Check sheet for the modelled part. Datum: model origin and axes. Units: mm. A direction names the side the tool comes from. Round coordinates to 2 decimals unless told otherwise and drop trailing zeros. Order: outer loops, then holes, each group sorted by start corner. A loop starts at its lowest first (then second) coordinate and runs counter-clockwise, first axis right, second up.
```python
from build123d import *

# Parameters (mm, degrees)
F0_W     = 21
F0_H     = 4
F0_R     = 26.5
F0_R_2   = 1
F1_DEPTH = 3
F2_DEPTH = 10
F4_R     = 1
F5_DEPTH = 37.501


with BuildPart() as f1:
    # F0 (on Front) → F1 (new body)
    with BuildSketch(Plane.XZ):
        with Locations((10.5, 9)):
            Rectangle(F0_W, F0_H)
        with Locations((-10.5, 9)):
            Rectangle(F0_W, F0_H)
        Circle(F0_R)
        with Locations((-16.334167, -16.334167)):
            Circle(F0_R_2, mode=Mode.SUBTRACT)
        with Locations((16.334167, -16.334167)):
            Circle(F0_R_2, mode=Mode.SUBTRACT)
        with Locations((-16.334167, 16.334167)):
            Circle(F0_R_2, mode=Mode.SUBTRACT)
        Polygon((21, 7), (0, 7), (-21, 7), (-21, 11), (0, 11), (21, 11), align=None, mode=Mode.SUBTRACT)
        with Locations((16.334167, 16.334167)):
            Circle(F0_R_2, mode=Mode.SUBTRACT)
    extrude(amount=F1_DEPTH)

    # F0 (on Front) → F2 (join)
    with BuildSketch(Plane.XZ):
        with Locations((10.5, 9)):
            Rectangle(F0_W, F0_H)
        with Locations((-10.5, 9)):
            Rectangle(F0_W, F0_H)
    extrude(amount=-F2_DEPTH)

    # F3: F1 across plane


with BuildPart() as f1_1:
    add(f1.part)
    add(f1.part.mirror(Plane.XY))

    # F4 (on face) → F5 (cut, through all)
    with BuildSketch(Plane.XY.offset(11)):
        with Locations((-12, 3)):
            Circle(F4_R)
        with Locations((12, 3)):
            Circle(F4_R)
    extrude(amount=-F5_DEPTH, mode=Mode.SUBTRACT)


solid = f1_1.part
```
Item 1: Go/stop test with flat-tipped pins: P1, Ø3, axis at x = 1.5, y = 2.5, coming from the +Z side; P2, Ø5, axis at x = 2.5, y = 6.5, coming from the -Z side; P3, Ø2, axis at y = 3, z = -9, coming from the +X side. Record where each tip stops, or that it passes through.
Answer:
P1: stops at z = 11
P2: stops at z = -11
P3: stops at x = 21
Item 2: Release check for a two-part mould opening along X. For faces 1 (the cylindrical face through (14.246, -1.479, 22.345)), 2 (the cylindrical face through (-15.41, -1.48, -16.72)), 3 (the flat face through (0, 5, -11)), 4 (the cylindrical face through (-13, 3, -9)) record: released by +X, released by -X, zero draft, split by the parting line, or undercut.
Answer:
face 1: split by the parting line
face 2: undercut
face 3: zero draft
face 4: undercut
Item 3: Sectioned sample at A-A (y = 7.25). Record the cut outline in (x, z), and give its area (3 significant figures).
Answer:
outline: (-21, -11) - (21, -11) - (21, -7) - (-21, -7) - close; (-21, 7) - (21, 7) - (21, 11) - (-21, 11) - close
area: 336 mm2
Item 4: Sectioned sample at C-C (x = -12). Record the cut outline in (y, z), and give its area (3 significant figures).
Answer:
outline: (-3, -23.63) - (0, -23.63) - (0, -11) - (2, -11) - (2, -7) - (0, -7) - (0, 7) - (2, 7) - (2, 11) - (0, 11) - (0, 23.63) - (-3, 23.63) - close; (4, -11) - (10, -11) - (10, -7) - (4, -7) - close; (4, 7) - (10, 7) - (10, 11) - (4, 11) - close
area: 206 mm2
Item 5: Sectioned sample at D-D (x = -3). Record the cut outline in (y, z), and give its area (3 significant figures).
Answer:
outline: (-3, -26.33) - (0, -26.33) - (0, -11) - (10, -11) - (10, -7) - (0, -7) - (0, 7) - (10, 7) - (10, 11) - (0, 11) - (0, 26.33) - (-3, 26.33) - close
area: 238 mm2
Item 6: Access from +Z, -Z, +X, -X, +Y, -Y to the whole of each face (thin tool, end or side, straight path). Record for faces 5 (the flat face through (21, 5, -9)), 6 (the flat face through (-21, 5, 9)), 7 (the flat face through (0, 5, 11)), 8 (the flat face through (0, 5, 7)), 9 (the flat face through (0, -3, 0)).
Answer:
face 5: +Z, -Z, +X, +Y
face 6: +Z, -Z, -X, +Y
face 7: +Z, +X, -X, +Y
face 8: +X, -X, +Y
face 9: +Z, -Z, +X, -X, -Y
Item 7: Sectioned sample at B-B (y = 3). Record the cut outline in (x, z), and give its area (3 significant figures).
Answer:
outline: (-21, -11) - (-13, -11) - (-13, -7) - (-21, -7) - close; (-21, 7) - (-13, 7) - (-13, 11) - (-21, 11) - close; (-11, -11) - (11, -11) - (11, -7) - (-11, -7) - close; (-11, 7) - (11, 7) - (11, 11) - (-11, 11) - close; (13, -11) - (21, -11) - (21, -7) - (13, -7) - close; (13, 7) - (21, 7) - (21, 11) - (13, 11) - close
area: 304 mm2
Item 8: Scan lines: line 1 along Z through (x, y) = (16.5, 2.5); line 2 along Y through (x, z) = (-12, 9.8); line 3 along Y through (x, z) = (-11, 18). Record each from-to range of solid material in increasing order.
Answer:
line 1: z = -11 to -7, 7 to 11
line 2: y = -3 to 2, 4 to 10
line 3: y = -3 to 0
